```python
from build123d import *

# Parameters (mm, degrees)
F0_W     = 100
F0_H     = 24
F0_R     = 10
F1_DEPTH = 24
F2_R     = 10
F3_DEPTH = 5
F5_D     = 3.3
F5_DEPTH = 14.1
F5_TIP   = 0.9914200214


with BuildPart() as f1:
    # F0 (on Right) → F1 (new body)
    with BuildSketch(Plane.YZ):
        Rectangle(F0_W, F0_H)
        with Locations((-30, 0)):
            Circle(F0_R, mode=Mode.SUBTRACT)
        with Locations((30, 0)):
            Circle(F0_R, mode=Mode.SUBTRACT)
    extrude(amount=F1_DEPTH)

    # F2 (on face) → F3 (cut)
    with BuildSketch(Plane(origin=(0, 0, 0), x_dir=(0, -1, 0), z_dir=(-1, 0, 0))):
        with BuildLine():
            ThreePointArc((-16.25, -12), (-12.9119925094, -6.408002809), (-11.75, 0))
            ThreePointArc((-11.75, 0), (-12.9119925094, 6.408002809), (-16.25, 12))
            Line((-16.25, 12), (-43.75, 12))
            ThreePointArc((-43.75, 12), (-48.25, 0), (-43.75, -12))
            Line((-43.75, -12), (-16.25, -12))
        make_face()
        with Locations((-30, 0)):
            Circle(F2_R, mode=Mode.SUBTRACT)
        with BuildLine():
            Line((43.75, 12), (16.25, 12))
            ThreePointArc((16.25, 12), (11.75, 0), (16.25, -12))
            Line((16.25, -12), (43.75, -12))
            ThreePointArc((43.75, -12), (47.0880074906, -6.408002809), (48.25, 0))
            ThreePointArc((48.25, 0), (47.0880074906, 6.408002809), (43.75, 12))
        make_face()
        with Locations((30, 0)):
            Circle(F2_R, mode=Mode.SUBTRACT)
    extrude(amount=-F3_DEPTH, mode=Mode.SUBTRACT)

    # F5
    with Locations(Plane(origin=(5, 0, 0), x_dir=(0, -1, 0), z_dir=(-1, 0, 0))):
        with Locations((-41.2583302492, 6.5), (-41.2583302492, -6.5), (-18.7416697508, 6.5), (-18.7416697508, -6.5), (18.7416697508, 6.5), (18.7416697508, -6.5), (41.2583302492, 6.5), (41.2583302492, -6.5)):
            Hole(F5_D / 2, depth=F5_DEPTH)
            with Locations((0, 0, -(F5_DEPTH + F5_TIP / 2))):  # 118° drill point
                Cone(0, F5_D / 2, F5_TIP, mode=Mode.SUBTRACT)


solid = f1.part
```
Source: CAD feature listing. Evaluate the final solid. Frame: model axes, mm. A direction names the side the tool comes from. Give positions to 0.01 mm unless a question says otherwise; leave off trailing zeros. Loops run counter-clockwise (first coordinate to the right, second up) from the corner with the lowest first, then second, coordinate; pieces in that order, holes last. Notation, with made-up numbers: M -7.75,70 L 36.25,70 A9 cw 36.25,76 Z; hole C 83.25,-21 d4. An arc over 180 degrees is marked long. Put each result on its own line as item: value.
Q1. Section B-B (x = 17.5). Count the separate pieces of the cut face and the enclosed holes in it, and give its area (3 significant figures).
Response values:
separate pieces: 1
enclosed holes: 10
area: 1,700 mm²
Q2. Reachability of faces 1 (the cylindrical face through (12.15, -19.1, 4.89)), 2 (the flat face through (24, -1, 0)) from +Z, -Z, +X, -X, +Y, -Y: full face, straight path, thin tool, end or side. Return the list, or none.
Response values:
face 1: -X
face 2: +Z, -Z, +X, +Y, -Y
Q3. Section A-A (y = 30). Return the cut outline in (x, z).
Response values:
outline: M 5,-12 L 24,-12 L 24,-10 L 5,-10 Z; M 5,10 L 24,10 L 24,12 L 5,12 Z
Q4. Mould query, pull axis Y, two halves, no side actions, for faces 3 (the flat face through (0, 0, 0)), 4 (the cylindrical face through (12.149, -39.734, -7.132)), 5 (the flat face through (12, 50, 0)). Classes: released by +Y, released by -Y, zero draft, split by the parting line, or undercut.
Response values:
face 3: zero draft
face 4: undercut
face 5: released by +Y
Q5. Section D-D (y = -35). Return the cut outline in (x, z).
Response values:
outline: M 5,-12 L 24,-12 L 24,-8.66 L 5,-8.66 Z; M 5,8.66 L 24,8.66 L 24,12 L 5,12 Z
Q6. Line query: probe 1 along Y at (x, z) = (18, -4); probe 2 along Z at (x, y) = (9, -17.5); probe 3 along Y at (x, z) = (16.75, 9.25). Output: solid intervals per line, ascending. Write a range as [from, to].
Response values:
probe 1: y = [-50, -39.17], [-20.83, 20.83], [39.17, 50]
probe 2: z = [-12, -7.59], [-5.41, 5.41], [7.59, 12]
probe 3: y = [-50, -33.8], [-26.2, 26.2], [33.8, 50]
Q7. Section C-C (z = -1.75). Return the cut outline in (x, y), and give its area (3 significant figures).
Response values:
outline: M 0,-50 L 24,-50 L 24,-39.85 L 5,-39.85 L 5,-48.17 L 0,-48.17 Z; M 0,-11.83 L 5,-11.83 L 5,-20.15 L 24,-20.15 L 24,20.15 L 5,20.15 L 5,11.83 L 0,11.83 Z; M 0,48.17 L 5,48.17 L 5,39.85 L 24,39.85 L 24,50 L 0,50 Z
area: 1,290 mm²
Q8. Pin query (flat end, axial travel): P1, Ø1, axis at y = -22, z = -7.5, coming from the -X side; P2, Ø3, axis at y = -41.26, z = -6.5, coming from the -X side. Return the tip coordinate at first contact, or that it passes through.
Response values:
P1: stops at x = 5
P2: stops at x = 19.19
